Could you check a few things on this drawing? It's one solid part, dimensions in mm from its lowest x, y, z. A direction names the side the tool comes from. Coordinates: 2 decimals unless noted, no trailing zeros. Write each loop counter-clockwise with the first axis right and the second up, starting at its lowest first coordinate (ties: lowest second). Pieces come first, ordered by that corner, then holes.
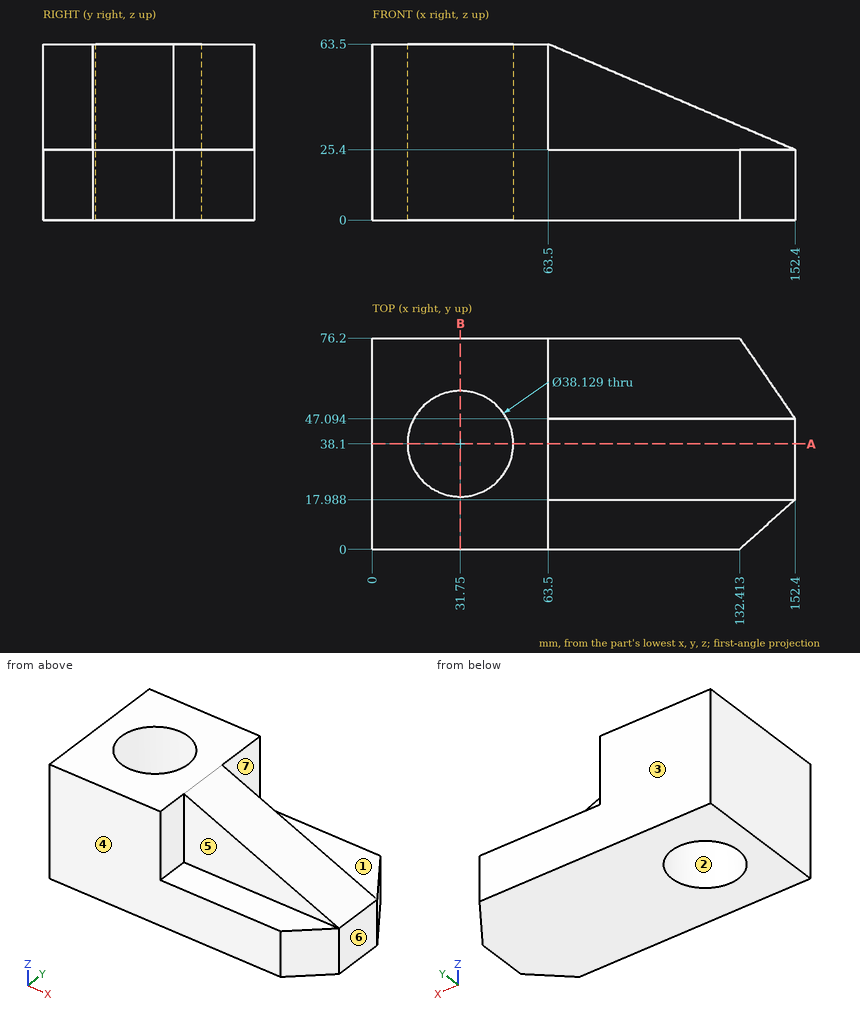
1) Will these pins go through, and if not, where does the flat tip stop? pin 1 (1.5 mm diameter, centred on x = 127, y = 17.5, fed in from +Z); pin 2 (6 mm diameter, centred on x = 73.5, z = 47, fed in from +Y); pin 3 (20 mm diameter, centred on x = 112, y = 12, fed in from +Z).
Values follow:
pin 1: stops at z = 36.53
pin 2: stops at y = 47.09
pin 3: stops at z = 46.15
2) We'd pull the mould along Y, two halves only. Please class the marked faces 1, 2, 3 and 4: pulls with the +Y half, pulls with the -Y half, needs draft (parallel to the pull), parting line crosses it, or undercut.
Values follow:
face 1: needs draft
face 2: undercut
face 3: pulls with the +Y half
face 4: pulls with the -Y half
3) On a 3-axis mill with a long thin cutter (end or side, diameter ignored), from which of +Z, -Z, +X, -X, +Y, -Y can I reach the whole of each face in a straight line? I mean the marked faces 5, 6 and 7. Say none if no direction works.
Values follow:
face 5: +Z, +X, -Y
face 6: +Z, -Z, +X, +Y, -Y
face 7: +Z, +X, +Y
4) Imagine slicing it at A-A on y = 38.1. Please give me the cut outline in (x, z) (1 decimal).
Values follow:
outline: (0, 0) - (12.7, 0) - (12.7, 63.5) - (0, 63.5) - close; (50.8, 0) - (152.4, 0) - (152.4, 25.4) - (63.5, 63.5) - (50.8, 63.5) - close
5) I need wall thicknesses on probe 1 along Y at (x, z) = (31, 47); probe 2 along Y at (x, z) = (31.75, 28) (1 decimal); probe 3 along X at (y, z) = (72.5, 59). Which ranges of each line are inside material? Lowest first, please.
Values follow:
probe 1: y = 0 to 19.05, 57.15 to 76.2
probe 2: y = 0 to 19, 57.2 to 76.2
probe 3: x = 0 to 63.5
6) Imagine slicing it at B-B on x = 31.75. Please give me the cut outline in (y, z) (1 decimal), then the cut area to 3 significant figures.
Values follow:
outline: (0, 0) - (19, 0) - (19, 63.5) - (0, 63.5) - close; (57.2, 0) - (76.2, 0) - (76.2, 63.5) - (57.2, 63.5) - close
area: 2,420 mm2
